The model under review builds one solid part; all positions refer to its coordinate system, in mm. A direction names the side the tool comes from. Round coordinates to 2 decimals unless told otherwise and drop trailing zeros. Loops run counter-clockwise (first coordinate to the right, second up) from the corner with the lowest first, then second, coordinate; pieces in that order, holes last. Notation, with made-up numbers: M 12,73.25 L 60,73.25 A15 cw 60,92.25 Z; hole C 87.25,28 d10. An arc over 180 degrees is marked long. Return JSON: item names as keys, results as strings. Group by question number.
Q1. Draft analysis for pull direction X (two halves, no side actions). For faces 4 (the face through (50.26, -24, 2.59)), 5 (the face through (1.5, -33, 7)), 6 (the face through (-1, -34.9, 4)), state which applies: pulls with the +X half, pulls with the -X half, needs draft (parallel to the pull), parting line crosses it, or undercut.
Q2. For faces 1 (the face through (45.38, -30.93, 4.06)), 2 (the face through (57.14, -25.8, 3.94)), 3 (the face through (-17, -33, 5.25)), list the 3-axis set-ups (+Z, -Z, +X, -X, +Y, -Y) from which the entire face can be reached by the end or side of a thin tool; tool diameter is ignored.
Q3. Consider section A-A (x = 30.5). State the section outline as (y, z) points.
Q4. Consider section D-D (y = 29.9). State the section outline as (x, z) points.
Q5. To check wall thickness, follow line 1 along Y through (x, z) = (-53, 4.75); line 2 along X through (y, z) = (14.5, 1.25); line 3 along Y through (x, z) = (-33.5, 4.5). State the ranges of each line that lie inside material, in increasing order.
Q6. Consider section C-C (y = 18). State the section outline as (x, z) points.
Q7. Consider section B-B (y = -30.1). State the section outline as (x, z) points.
Q8. Clearance check with flat-ended pins moving along their axes: pin 1 Ø4 at (x, y) = (50.5, 20.5) entering from +Z; pin 2 Ø2.5 at (y, z) = (9.5, 3.5) entering from -X; pin 3 Ø0.8 at (y, z) = (-34, 6.5) entering from +X. State where each tip first meets the part, or that it passes through.
from build123d import *

# Parameters (mm, degrees)
FRAMEOUTSIDE_W                    = 98.8
FRAMEOUTSIDE_H                    = 69.8
FRAME_HEIGHT_8_DEPTH              = 8
OUTSIDE_R6P4_R                    = 6.4
FRAMEINSIDE_W                     = 92.8
FRAMEINSIDE_H                     = 63.8
OPEN_THROUGH_FRAME_DEPTH          = 8.3
INSIDE_R3P4_R                     = 3.4
FOUR_CORNER_EARS_R2_PITCH110X80_R = 1.6
INTEGRAL_EARS_4X3P2_DEPTH         = 8
OPEN_TOP_CABLE_RELIEFS_START      = 5.25
PLUG_CLEARANCE_PROFILES_W         = 12
PLUG_CLEARANCE_PROFILES_H         = 8
PLUG_CLEARANCE_PROFILES_W_2       = 9.6
PLUG_CLEARANCE_PROFILES_W_3       = 8.5
PLUG_CLEARANCE_PROFILES_H_2       = 19.2
PLUG_CLEARANCE_PROFILES_H_3       = 16.6
OPEN_TOP_CABLE_RELIEFS_DEPTH      = 3.25
FILLET_1_R                        = 3


with BuildPart() as part:
    # FrameOutside → Frame_Height_8 (new body)
    with BuildSketch(Plane.XY):
        Rectangle(FRAMEOUTSIDE_W, FRAMEOUTSIDE_H)
    extrude(amount=FRAME_HEIGHT_8_DEPTH)

    # Outside_R6p4
    outside_r6p4_edges = [part.edges().sort_by_distance(p)[0] for p in [
        (49.4, -34.9, 4),
        (-49.4, -34.9, 4),
        (-49.4, 34.9, 4),
        (49.4, 34.9, 4),
    ]]
    fillet(outside_r6p4_edges, radius=OUTSIDE_R6P4_R)

    # FrameInside → Open_Through_Frame (cut)
    with BuildSketch(Plane.XY):
        Rectangle(FRAMEINSIDE_W, FRAMEINSIDE_H)
    extrude(amount=OPEN_THROUGH_FRAME_DEPTH, mode=Mode.SUBTRACT)

    # Inside_R3p4
    inside_r3p4_edges = [part.edges().sort_by_distance(p)[0] for p in [
        (46.4, -31.9, 4),
        (46.4, 31.9, 4),
        (-46.4, 31.9, 4),
        (-46.4, -31.9, 4),
    ]]
    fillet(inside_r3p4_edges, radius=INSIDE_R3P4_R)

    # Four_Corner_Ears_R2_Pitch110x80 → Integral_Ears_4x3p2 (add)
    # profile 1 of 4: a face of its own
    with BuildSketch(Plane.XY):
        Polygon((43, 34.9), (58, 34.9), (58, 24.9), (49.4, 24.9), align=None)
        with Locations((54, 29.9)):
            Circle(FOUR_CORNER_EARS_R2_PITCH110X80_R, mode=Mode.SUBTRACT)
    # profile 2 of 4: a face of its own
    with BuildSketch(Plane.XY):
        Polygon((43, -34.9), (58, -34.9), (58, -24.9), (49.4, -24.9), align=None)
        with Locations((54, -30.1)):
            Circle(FOUR_CORNER_EARS_R2_PITCH110X80_R, mode=Mode.SUBTRACT)
    # profile 3 of 4: a face of its own
    with BuildSketch(Plane.XY):
        Polygon((-43, -34.9), (-58, -34.9), (-58, -24.9), (-49.480769769, -24.9), align=None)
        with Locations((-53, -30.1)):
            Circle(FOUR_CORNER_EARS_R2_PITCH110X80_R, mode=Mode.SUBTRACT)
    # profile 4 of 4: a face of its own
    with BuildSketch(Plane.XY):
        Polygon((-43, 34.9), (-58, 34.9), (-58, 24.9), (-49.4, 24.9), align=None)
        with Locations((-53, 29.9)):
            Circle(FOUR_CORNER_EARS_R2_PITCH110X80_R, mode=Mode.SUBTRACT)
    extrude(amount=INTEGRAL_EARS_4X3P2_DEPTH)

    # Plug_Clearance_Profiles → Open_Top_Cable_Reliefs (cut)
    with BuildSketch(Plane.XY.offset(OPEN_TOP_CABLE_RELIEFS_START)):
        with Locations((-31.3, -35)):
            Rectangle(PLUG_CLEARANCE_PROFILES_W, PLUG_CLEARANCE_PROFILES_H)
        with Locations((-16.7, -35)):
            Rectangle(PLUG_CLEARANCE_PROFILES_W_2, PLUG_CLEARANCE_PROFILES_H)
        with Locations((-3.3, -35)):
            Rectangle(PLUG_CLEARANCE_PROFILES_W_2, PLUG_CLEARANCE_PROFILES_H)
        with Locations((49.75, -17.8)):
            Rectangle(PLUG_CLEARANCE_PROFILES_W_3, PLUG_CLEARANCE_PROFILES_H_2)
        with Locations((49.75, 1.1)):
            Rectangle(PLUG_CLEARANCE_PROFILES_W_3, PLUG_CLEARANCE_PROFILES_H_3)
        with Locations((49.75, 19)):
            Rectangle(PLUG_CLEARANCE_PROFILES_W_3, PLUG_CLEARANCE_PROFILES_H_3)
    extrude(amount=OPEN_TOP_CABLE_RELIEFS_DEPTH, mode=Mode.SUBTRACT)

    # 圆角1
    # the kernel refuses this fillet: 3 mm, written as the material it adds along each edge
    with BuildSketch(Plane(origin=(-49.4, 24.9, 0), x_dir=(0, -1, 0), z_dir=(0, 0, 1))) as fillet_1_piece_1:
        with BuildLine():
            CenterArc((FILLET_1_R, -FILLET_1_R), FILLET_1_R, 90, 90)
            Line((0, -FILLET_1_R), (0, 0))
            Line((0, 0), (FILLET_1_R, 0))
        make_face()
    extrude(amount=8)
    with BuildSketch(Plane(origin=(49.4, -24.9, 0), x_dir=(1, 0, 0), z_dir=(0, 0, 1)), Plane(origin=(49.4, 24.9, 0), x_dir=(0, -1, 0), z_dir=(0, 0, 1))) as fillet_1_piece_2:
        with BuildLine():
            CenterArc((FILLET_1_R, FILLET_1_R), FILLET_1_R, 180, 90)
            Line((0, FILLET_1_R), (0, 0))
            Line((0, 0), (FILLET_1_R, 0))
        make_face()
    extrude(amount=5.25)
    # the kernel refuses this fillet: 3 mm, written as the material it takes off along each edge
    with BuildSketch(Plane(origin=(-58, 34.9, -7.5), x_dir=(1, 0, 0), z_dir=(0, 0, 1)), Plane(origin=(-58, 24.9, -7.5), x_dir=(0, 1, 0), z_dir=(0, 0, 1)), Plane(origin=(-58, -24.9, -7.5), x_dir=(1, 0, 0), z_dir=(0, 0, 1)), Plane(origin=(-58, -34.9, -7.5), x_dir=(0, 1, 0), z_dir=(0, 0, 1)), Plane(origin=(58, -24.9, -7.5), x_dir=(0, -1, 0), z_dir=(0, 0, 1)), Plane(origin=(58, -34.9, -7.5), x_dir=(-1, 0, 0), z_dir=(0, 0, 1)), Plane(origin=(58, 24.9, -7.5), x_dir=(-1, 0, 0), z_dir=(0, 0, 1)), Plane(origin=(58, 34.9, -7.5), x_dir=(0, -1, 0), z_dir=(0, 0, 1))) as fillet_1_2_piece_1:
        with BuildLine():
            CenterArc((FILLET_1_R, -FILLET_1_R), FILLET_1_R, 90, 90)
            Line((0, -FILLET_1_R), (0, 0))
            Line((0, 0), (FILLET_1_R, 0))
        make_face()
    extrude(amount=23, mode=Mode.SUBTRACT)
    with BuildSketch(Plane(origin=(-49.480769769, -24.9, -1.937361077), x_dir=(0.5438533962151781, -0.8391802448968972, 0), z_dir=(0, 0, 1))) as fillet_1_2_piece_2:
        with BuildLine():
            CenterArc((2.096084574, -2.281878246), FILLET_1_R, 130.480576978, 16.573079502)
            Line((-0.421456161, -0.650318057), (0, 0))
            Line((0, 0), (0.148513864, 0))
        make_face()
    extrude(amount=11.874722155, mode=Mode.SUBTRACT)


solid = part.part
Values:
{
 "1": {"face 4": "pulls with the +X half", "face 5": "undercut", "face 6": "needs draft"},
 "2": {"face 1": "+Z, -Z", "face 2": "+Z, -Z, +X", "face 3": "+Z, -Y"},
 "3": {"outline": "M -34.9,0 L -31.9,0 L -31.9,8 L -34.9,8 Z; M 31.9,0 L 34.9,0 L 34.9,8 L 31.9,8 Z"},
 "4": {"outline": "M -58,0 L -54.6,0 L -54.6,8 L -58,8 Z; M -51.4,0 L -46.1,0 L -46.1,8 L -51.4,8 Z; M 46.1,0 L 52.4,0 L 52.4,8 L 46.1,8 Z; M 55.6,0 L 58,0 L 58,8 L 55.6,8 Z"},
 "5": {"line 1": "y = -34.9 to -31.7, -28.5 to -24.9, 24.9 to 28.3, 31.5 to 34.9", "line 2": "x = -49.4 to -46.4, 46.4 to 49.4", "line 3": "y = -34.9 to -31.9, 31.9 to 34.9"},
 "6": {"outline": "M -49.4,0 L -46.4,0 L -46.4,8 L -49.4,8 Z; M 46.4,0 L 49.4,0 L 49.4,5.25 L 46.4,5.25 Z"},
 "7": {"outline": "M -58,0 L -54.6,0 L -54.6,8 L -58,8 Z; M -51.4,0 L -46,0 L -46,8 L -51.4,8 Z; M 46,0 L 52.4,0 L 52.4,8 L 46,8 Z; M 55.6,0 L 58,0 L 58,8 L 55.6,8 Z"},
 "8": {"pin 1": "stops at z = 5.25", "pin 2": "stops at x = -49.4", "pin 3": "stops at x = 57.47"}
}
